Could you check a few things on this model? Use its own coordinates, in mm. A direction names the side the tool comes from. Give positions to 0.01 mm unless a question says otherwise; leave off trailing zeros. Loops run counter-clockwise (first coordinate to the right, second up) from the corner with the lowest first, then second, coordinate; pieces in that order, holes last. Notation, with made-up numbers: M 83.25,-18 L 96.25,-18 A19 ccw 96.25,10 Z; hole C 46.25,50.25 d3. An arc over 180 degrees is marked long. Answer in a Markdown table with one row per item. Add a question column.
1. Thinking about a two-plate mould opening in Y: for faces 6 (the flat face through (-7, -20.35, -54)), 7 (the flat face through (-7, 5, 12.7)), 8 (the flat face through (-5, 13, 3.431)), which applies, released by +Y, released by -Y, zero draft, split by the parting line, or undercut?
2. If we section it at B-B on x = -3.5: List the corners of the cut face in (y, z) for me, then the cut area to 3 significant figures.
3. If we section it at D-D on x = 21: List the corners of the cut face in (y, z) for me, then the cut area to 3 significant figures.
4. I'm going to push flat-ended pins straight in: pin 1 Ø6.5 at (y, z) = (0, 8.5) entering from +X; pin 2 Ø14 at (y, z) = (7.5, 3.5) entering from -X; pin 3 Ø4 at (x, y) = (1.5, 7.5) entering from -Z. Where does each tip first touch, or does it pass through?
5. Which directions (+Z, -Z, +X, -X, +Y, -Y) give clear straight access to the entire face, cutting with the end or side of a thin tool? Please do faces 1 (the flat face through (-7, -7.65, -61)), 2 (the flat face through (-56.635, 5, 6)), 3 (the flat face through (-7, 30.45, 6)), 4 (the flat face through (-5.124, 9.312, 1.739)), 5 (the flat face through (44.965, 5, 6)).
6. I need wall thicknesses on line 1 along Y through (x, z) = (31, -92); line 2 along Z through (x, y) = (-3, 21.5); line 3 along Z through (x, y) = (-34, -10). Which ranges of each line are inside material? Lowest first, please. Write a range as from..to.
7. If we section it at C-C on z = -71: List the corners of the cut face in (x, y) for me, then the cut area to 3 significant figures.
8. If we section it at A-A on y = -11: List the corners of the cut face in (x, z) for me.
```python
from build123d import *

# Parameters (mm, degrees)
F0_W     = 101.6
F0_H     = 50.8
F1_DEPTH = 12.7
F3_DEPTH = 101.6
F5_DEPTH = 12.7


with BuildPart() as f1:
    # F0 (on Top) → F1 (new body)
    with BuildSketch(Plane.XY):
        with Locations((-5.834938, 5.050136)):
            Rectangle(F0_W, F0_H)
    extrude(amount=F1_DEPTH)

    # F2 (on face) → F3 (cut)
    with BuildSketch(Plane.YZ.offset(44.965062)):
        Polygon((7.780036, 0), (11.336036, 0), (14.358213, 3.43069), (10.802213, 3.43069), align=None)
    extrude(amount=-F3_DEPTH, mode=Mode.SUBTRACT)

    # F4 (on face) → F5 (join)
    with BuildSketch(Plane.XZ.offset(20.349864)):
        with BuildLine():
            ThreePointArc((-56.634938, 0), (-33.640743, -117.969016), (66.378369, -51.323695))
            ThreePointArc((66.378369, -51.323695), (60.810383, -23.517889), (44.965062, 0))
            Line((44.965062, 0), (-56.634938, 0))
        make_face()
    extrude(amount=-F5_DEPTH)


solid = f1.part
```
Results:
| question | item | result |
|---|---|---|
| 1 | face 6 | released by -Y |
| 1 | face 7 | zero draft |
| 1 | face 8 | undercut |
| 2 | outline | M -20.35,-123.5 L -7.65,-123.5 L -7.65,0 L 7.78,0 L 10.8,3.43 L 14.36,3.43 L 11.34,0 L 30.45,0 L 30.45,12.7 L -20.35,12.7 Z |
| 2 | area | 2,200 mm2 |
| 3 | outline | M -20.35,-118.37 L -7.65,-118.37 L -7.65,0 L 7.78,0 L 10.8,3.43 L 14.36,3.43 L 11.34,0 L 30.45,0 L 30.45,12.7 L -20.35,12.7 Z |
| 3 | area | 2,140 mm2 |
| 4 | pin 1 | x = 44.97 |
| 4 | pin 2 | x = -56.63 |
| 4 | pin 3 | z = 0 |
| 5 | face 1 | -Z, +X, -X, +Y |
| 5 | face 2 | +Z, -X, +Y, -Y |
| 5 | face 3 | +Z, -Z, +X, -X, +Y |
| 5 | face 4 | -Z, +X, -X |
| 5 | face 5 | +Z, +X, +Y, -Y |
| 6 | line 1 | -20.35..-7.65 |
| 6 | line 2 | 0..12.7 |
| 6 | line 3 | -117.82..12.7 |
| 7 | outline | M -75.32,-20.35 L 63.65,-20.35 L 63.65,-7.65 L -75.32,-7.65 Z |
| 7 | area | 1,760 mm2 |
| 8 | outline | M -56.63,0 A72.21 ccw long 66.38,-51.32 A72.21 ccw 44.97,0 L 44.97,12.7 L -56.63,12.7 Z |
